For this review, take the finished solid that the model builds, in its own axes (mm). Face numbers are marked on the shaded views. A direction names the side the tool comes from. Coordinates: 2 decimals unless noted, no trailing zeros. Loops run counter-clockwise (first coordinate to the right, second up) from the corner with the lowest first, then second, coordinate; pieces in that order, holes last.
```python
from build123d import *

# Parameters (mm, degrees)
PAD_DEPTH              = 55
PAD003_DEPTH           = 2
SKETCH005_W            = 5
SKETCH005_H            = 55
PAD004_DEPTH           = 9.5
LINEARPATTERN_COUNT    = 2
LINEARPATTERN_PITCH    = 11.5
PAD005_DEPTH           = 3
LINEARPATTERN001_COUNT = 3
LINEARPATTERN001_PITCH = 25


with BuildPart() as part:
    # Sketch004 → Pad (new body)
    with BuildSketch(Plane.XY):
        Polygon((0, -5), (-25, -5), (-25, 53), (-20, 53), (-20, 15), (-8, 15), (-8, 0), (0, 0), align=None)
    extrude(amount=-PAD_DEPTH)

    # Sketch (on Face8 of Pad) → Pad003 (join)
    with BuildSketch(Plane.YZ):
        Polygon((-5, -55), (0, -55), (0, -51), (2.1, -51), (2.1, -55), (8.1, -55), (8.1, -42), (0, -42), (0, -19), (2.1, -19), (2.1, -23), (8.1, -23), (8.1, -10), (0, -10), (0, 0), (-5, 0), align=None)
    pad003 = extrude(amount=PAD003_DEPTH)

    # Sketch005 (on Face8 of Pad003) → Pad004 (join)
    with BuildSketch(Plane.YZ.offset(2)):
        with Locations((-2.5, -27.5)):
            Rectangle(SKETCH005_W, SKETCH005_H)
    extrude(amount=PAD004_DEPTH)

    # LinearPattern: Pad003 ×2
    with Locations(*[(i * LINEARPATTERN_PITCH, 0, 0) for i in range(1, LINEARPATTERN_COUNT)]):
        add(pad003)

    # Sketch006 (on DatumPlane) → Pad005 (join)
    with BuildSketch(Plane.XZ):
        Polygon((-25, -12.5), (-30, -12.5), (-30, -42.5), (-25, -42.5), (-25, -38.5), (-28, -38.5), (-28, -16.5), (-25, -16.5), align=None)
    pad005 = extrude(amount=PAD005_DEPTH)

    # LinearPattern001: Pad005 ×3
    with Locations(*[(0, i * LINEARPATTERN001_PITCH, 0) for i in range(1, LINEARPATTERN001_COUNT)]):
        add(pad005)


solid = part.part
```
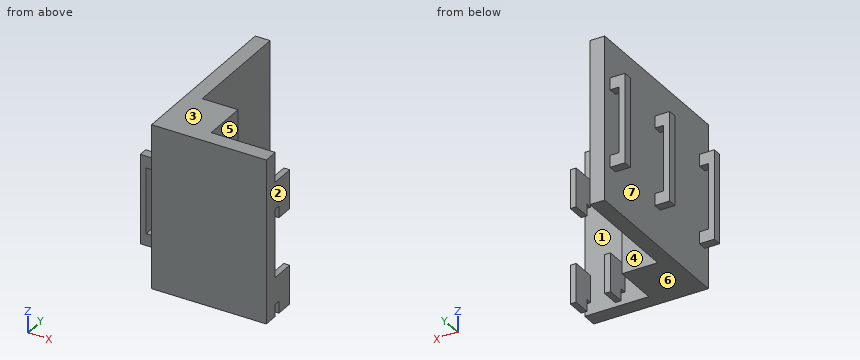
Q1. Consider section C-C (z = -34.5). State the section outline as (x, y) points, then the cut area to 4 significant figures.
Q2. Consider section D-D (x = 3.5). State the section outline as (y, z) points.
Q3. Consider section B-B (y = 3). State the section outline as (x, z) points, then the cut area to 3 significant figures.
Q4. Wall thickness on probe 1 along X at (y, z) = (24.5, -29.5); probe 2 along Z at (x, y) = (-26.5, 24); probe 3 along Y at (x, z) = (7, -7.5): over which ranges is each line inside the solid? List them lowest first.
Q5. Consider section A-A (x = -26.5). State the section outline as (y, z) points, then the cut area to 3 significant figures.
Q6. For pin 1 Ø1.5 at (x, y) = (-9, 15) entering from +Z; pin 2 Ø2.5 at (x, z) = (-28.5, -25) entering from +Y; pin 3 Ø5.5 at (x, z) = (-28.5, -27.5) entering from -Y; pin 4 Ø1.5 at (x, z) = (-8, -38) entering from +Y, all flat-tipped, find the tip position at first contact; note any pin that passes through.
Q7. Machinability: for the marked faces 4, 5, 6 and 7, which of the approach directions +Z, -Z, +X, -X, +Y, -Y give a long, thin tool a straight path to every point of the face, cutting with its end or side? Answer none if there is none.
Q8. The part is to be moulded in two halves that separate along X. For the marked faces 1, 2 and 3, say which applies: +X half, -X half, draft (parallel to the pull), parting line (faces both ways), or undercut.
Model answer:
1. outline: (-30, -3) - (-28, -3) - (-28, 0) - (-30, 0) - close; (-30, 22) - (-28, 22) - (-28, 25) - (-30, 25) - close; (-30, 47) - (-28, 47) - (-28, 50) - (-30, 50) - close; (-25, -5) - (13.5, -5) - (13.5, 0) - (-8, 0) - (-8, 15) - (-20, 15) - (-20, 53) - (-25, 53) - close
1. area: 655.5 mm2
2. outline: (-5, -55) - (0, -55) - (0, 0) - (-5, 0) - close
3. outline: (-25, -55) - (-8, -55) - (-8, 0) - (-25, 0) - close; (0, -55) - (2, -55) - (2, -42) - (0, -42) - close; (0, -23) - (2, -23) - (2, -10) - (0, -10) - close; (11.5, -55) - (13.5, -55) - (13.5, -42) - (11.5, -42) - close; (11.5, -23) - (13.5, -23) - (13.5, -10) - (11.5, -10) - close
3. area: 1,040 mm2
4. probe 1: x = -30 to -28, -25 to -20
4. probe 2: z = -42.5 to -38.5, -16.5 to -12.5
4. probe 3: y = -5 to 0
5. outline: (-3, -42.5) - (0, -42.5) - (0, -38.5) - (-3, -38.5) - close; (-3, -16.5) - (0, -16.5) - (0, -12.5) - (-3, -12.5) - close; (22, -42.5) - (25, -42.5) - (25, -38.5) - (22, -38.5) - close; (22, -16.5) - (25, -16.5) - (25, -12.5) - (22, -12.5) - close; (47, -42.5) - (50, -42.5) - (50, -38.5) - (47, -38.5) - close; (47, -16.5) - (50, -16.5) - (50, -12.5) - (47, -12.5) - close
5. area: 72.0 mm2
6. pin 1: stops at z = 0
6. pin 2: stops at y = 50
6. pin 3: stops at y = -3
6. pin 4: stops at y = 15
7. face 4: +Z, -Z, +X, +Y
7. face 5: +Z, -Z, +Y
7. face 6: -Z, +X, -X, +Y, -Y
7. face 7: none
8. face 1: undercut
8. face 2: +X half
8. face 3: draft
